For this review, take the finished solid that the model builds, in its own axes (mm). A direction names the side the tool comes from. Give positions to 0.01 mm unless a question says otherwise; leave off trailing zeros. Loops run counter-clockwise (first coordinate to the right, second up) from the corner with the lowest first, then second, coordinate; pieces in that order, holes last.
Autodesk Inventor part; units mm, degrees
ref_plane "YZ Plane" through (0, 0, 0) normal (1, 0, 0) x (0, 1, 0)
ref_plane "XZ Plane" through (0, 0, 0) normal (0, 1, 0) x (-1, 0, 0)
ref_plane "XY Plane" through (0, 0, 0) normal (0, 0, 1) x (1, 0, 0)
sketch "Sketch1" plane through (0, 0, 0) normal (0, 1, 0) x (-1, 0, 0)
  line L0 (0, 0) -> (0, -60)
  line L1 (0, -60) -> (10, -60)
  line L2 (10, -60) -> (10, 0)
  line L3 (10, 0) -> (0, 0)
  line L4 (10, -60) -> (10, -58)
  line L5 (10, -58) -> (0, -58)
  line L6 (10, -58) -> (8, -58)
  line L7 (0, 0) -> (2, 0)
  line L8 (2, 0) -> (2, -2)
  line L9 (2, -2) -> (0, -2)
  line L10 (0, -2) -> (0, 0)
  line L11 (2, -2) -> (8, -2)
  line L12 (8, -2) -> (8, -58)
  line L13 (8, -58) -> (2, -58)
  line L14 (2, -58) -> (2, -2)
  line L15 (10, 0) -> (10, -10)
  line L16 (10, -10) -> (0, -10)
  line L17 (8, -10) -> (8, -18)
  line L18 (8, -18) -> (2, -18)
  line L19 (2, -18) -> (1, -18)
  point P0 (2, -10)
  dimension "d0" = 60
  dimension "d1" = 10
  dimension "d2" = 2
  dimension "d3" = 2
  dimension "d4" = 2
  dimension "d5" = 2
  dimension "d8" = 10
  dimension "d29" = 8
extrude "Extrusion1" add sketch "Sketch1" along normal blind 10 contours L3 L8 L9 L0 | L9 L14 L16 L0 | L3 L2 L16 L12 L11 L8 | L16 L14 L5 L0 | L11 L12 L16 L14 | L5 L2 L1 L0 | L2 L5 L12 L16
fillet "Fillet1" radius 5 2 edges at (-5, 10, 0) (-5, 0, 0)
sketch "Sketch2" plane through (0, 0, -60) normal (1, 0, 0) x (0, 0, -1)
  arc A0 (-55, 10) -> (-55, 0) centre (-55, 5) ccw
  line L0 (-55, 10) -> (-55, 0)
  circle A1 centre (-55, 5) radius 1.1
  point P0 (-60, 0)
  dimension "d10" = 2.2
extrude "Extrusion2" cut sketch "Sketch2" against normal through all contours A1 L0 | L0 A1
sketch "Sketch3" plane through (0, 0, -60) normal (1, 0, 0) x (0, 0, -1)
  circle A0 centre (-55, 5) radius 1.1
  line L0 (-55, 5) -> (-34.322, 5)
  circle A1 centre (-34.322, 5) radius 1.1
  point P0 (-60, 0)
  dimension "d13" = 20.678
  dimension "d53" = 2.2
extrude "Extrusion3" cut sketch "Sketch3" against normal through all contours A1
sketch "Sketch5" plane through (0, 10, 0) normal (0, 1, 0) x (1, 0, 0)
  line L0 (0, 26.778) -> (0, 24.578)
  line L1 (0, 25.678) -> (0, 37.678)
  line L2 (0, 37.678) -> (-10, 37.678)
  line L3 (-10, 60) -> (-10, 5)
  line L4 (-10, 37.678) -> (-10, 39.678)
  line L5 (-10, 39.678) -> (0, 39.678)
  line L6 (0, 5) -> (0, 60)
  line L7 (0, 39.678) -> (0, 41.678)
  line L8 (0, 41.678) -> (-10, 41.678)
  line L9 (-10, 39.678) -> (-10, 41.678)
  line L10 (0, 37.678) -> (0, 47.678)
  line L11 (0, 47.678) -> (-10, 47.678)
  line L12 (-10, 60) -> (-10, 5)
  point P0 (0, 0)
  point P1 (0, 41.678)
  dimension "d17" = 12
  dimension "d18" = 2
  dimension "d19" = 2
  dimension "d22" = 10
extrude "Extrusion4" add sketch "Sketch5" against normal blind 10
sketch "Sketch6" plane through (0, 10, 0) normal (0, 1, 0) x (1, 0, 0)
  line L0 (-10, 60) -> (0, 60)
  line L1 (0, 60) -> (0, 50.678)
  line L2 (0, 50.678) -> (-10, 50.678)
  line L3 (-10, 50.678) -> (-10, 60)
  line L4 (-10, 60) -> (-10, 47.678)
  line L5 (-10, 47.678) -> (0, 47.678)
  line L6 (-2, 47.678) -> (-8, 47.678)
  line L7 (0, 47.678) -> (0, 50.678)
  line L8 (0, 5) -> (0, 60)
  point P0 (0, 0)
extrude "Extrusion5" cut sketch "Sketch6" against normal blind 10
sketch "Sketch7" plane through (0, 5, -5) normal (1, 0, 0) x (0, 0, -1)
  line L0 (42.678, 5) -> (0, 5)
  circle A0 centre (37.678, 0) radius 1.1
  line L1 (5, 5) -> (32.678, 5)
  line L2 (37.678, 5) -> (37.678, -5)
  point P0 (-5, -5)
  point P1 (40.678, 5)
  point P2 (40.678, -5)
  point P3 (45.678, 5)
extrude "Extrusion6" cut sketch "Sketch7" against normal through all
sketch "Sketch8" plane through (0, 10, 0) normal (0, 1, 0) x (1, 0, 0)
  line L0 (0, 26.778) -> (0, 24.578)
  line L1 (0, 25.678) -> (-8, 25.678)
  line L2 (-8, 26.778) -> (-8, 24.578)
  line L3 (0, 25.678) -> (0, 17.678)
  line L4 (0, 5) -> (0, 47.678)
  line L5 (0, 17.678) -> (-2, 17.678)
  line L6 (-2, 37.678) -> (-2, 10)
  line L7 (-2, 17.678) -> (-1, 17.678)
  line L8 (-1, 17.678) -> (-1, 33.678)
  line L9 (-1, 33.678) -> (-2, 33.678)
  line L10 (-2, 33.678) -> (-9, 33.678)
  line L11 (-9, 33.678) -> (-9, 17.678)
  line L12 (-9, 17.678) -> (-2, 17.678)
  line L13 (-9, 33.678) -> (-9.25, 33.678)
  line L14 (-9.25, 33.678) -> (-9.25, 17.678)
  line L15 (-9.25, 17.678) -> (-9, 17.678)
  line L16 (-1, 17.678) -> (-0.75, 17.678)
  line L17 (-0.75, 17.678) -> (-0.75, 33.678)
  line L18 (-0.75, 33.678) -> (-1, 33.678)
  point P0 (0, 0)
  point P1 (0, 45.678)
  point P2 (0, 50.678)
  dimension "d30" = 8
  dimension "d31" = 16
  dimension "d32" = 7
  dimension "d50" = 0.25
  dimension "d51" = 0.25
extrude "Extrusion7" cut sketch "Sketch8" against normal blind 10 contours L17 L5 L8 L1 | L1 L8 L18 L17 | L8 L5 L6 L1 | L1 L6 L9 L8 | L6 L12 L11 L10 | L11 L15 L14 L13
fillet "Fillet3" radius 5 2 edges at (-5, 10, -47.678) (-5, 0, -47.678)
chamfer "Chamfer2" distance 1.25 angle 45 4 edges at (-9.25, 5, -17.678) (-9.25, 5, -33.678) (-0.75, 5, -17.678) (-0.75, 5, -33.678)
properties part number "mid"
Item 1: Take a section at B-B on x = -3.5. State how many separate pieces and enclosed holes the cut face has, and give its area (3 significant figures).
Answer:
separate pieces: 2
enclosed holes: 2
area: 171 mm2
Item 2: For L1, parallel to Z at x = -0.2, y = 5; L2, parallel to Y at x = -7.75, z = -5; L3, parallel to X at y = 5.5, z = -31, list the stretches that pass through material, from the lowest coordinate up.
Answer:
L1: z = -47.68 to -43.78, -41.58 to -26.78, -24.58 to -6.1, -3.9 to 0
L2: y = 0 to 3.9, 6.1 to 10
L3: x = -10 to -9.25, -0.75 to 0
Item 3: The part is to be moulded in two halves that separate along Z. For faces 3 (the cylindrical face through (-4.93, 1.426, -46.175)), 4 (the flat face through (-2, 5, -14)), 5 (the flat face through (-8, 5, -14)), 6 (the cylindrical face through (-5, 2, -1)), say which applies: released by +Z, released by -Z, zero draft, split by the parting line, or undercut.
Answer:
face 3: released by -Z
face 4: undercut
face 5: undercut
face 6: released by +Z
Item 4: Take a section at C-C on z = -19.5. Give the boundary of the cut face in (x, y), and give its area (3 significant figures).
Answer:
outline: (-10, 0) - (-9.25, 0) - (-9.25, 10) - (-10, 10) - close; (-0.75, 0) - (0, 0) - (0, 10) - (-0.75, 10) - close
area: 15.0 mm2
Item 5: Take a section at A-A on z = -34.5. Give the boundary of the cut face in (x, y), and give its area (3 significant figures).
Answer:
outline: (-10, 0) - (-8, 0) - (-8, 10) - (-10, 10) - close; (-2, 0) - (0, 0) - (0, 10) - (-2, 10) - close
area: 40.0 mm2
Item 6: Clearance check with flat-ended pins moving along their axes: pin 1 Ø2 at (y, z) = (5, -25.678) entering from +X; pin 2 Ø5 at (x, y) = (-6, 4.5) entering from +Z; pin 3 Ø2 at (x, y) = (-6.5, 1.5) entering from +Z; pin 4 Ø2 at (x, y) = (-8.5, 8) entering from +Z. State where each tip first meets the part, or that it passes through.
Answer:
pin 1: passes through
pin 2: stops at z = 0
pin 3: stops at z = -0.67
pin 4: stops at z = -0.42
Item 7: Tool access review of faces 1 (the flat face through (-8, 5, -36)), 2 (the cylindrical face through (-5, 8, -1)): name each direction out of +Z, -Z, +X, -X, +Y, -Y from which nothing blocks a thin tool from reaching the whole face with its end or side.
Answer:
face 1: +Y, -Y
face 2: +Z, +X, -X, +Y
